Design review of the part built by this model. Coordinates are the model's own, in mm. A direction names the side the tool comes from. Coordinates: 2 decimals unless noted, no trailing zeros. Write each loop counter-clockwise with the first axis right and the second up, starting at its lowest first coordinate (ties: lowest second). Pieces come first, ordered by that corner, then holes.
Q1. For pin 1 Ø5 at (y, z) = (-15, 40.5) entering from +X; pin 2 Ø4 at (x, z) = (-8.5, 45) entering from +Y; pin 3 Ø4 at (y, z) = (-9.06, 89) entering from +X, all flat-tipped, find the tip position at first contact; note any pin that passes through.
Q2. The part is to be moulded in two halves that separate along Z. For faces 1 (the flat face through (-12, -16.564, 48)), 2 (the cylindrical face through (-11.62, -15.82, 87.57)), say which applies: released by +Z, released by -Z, zero draft, split by the parting line, or undercut.
Q3. Take a section at D-D, the plane y = -2.75. Write out the cut boundary in (x, z), plus the area to 3 significant figures.
Q4. Take a section at B-B, the plane y = -9.25. Write out the cut boundary in (x, z).
Q5. For L1, parallel to Y at x = -18.95, z = 89; L2, parallel to X at y = -16, z = 89; L3, parallel to Y at x = -5.75, z = 57.5, list the stretches that pass through material, from the lowest coordinate up.
Q6. Take a section at A-A, the plane z = 7.5. Write out the cut boundary in (x, y).
Q7. Take a section at C-C, the plane x = -15.5. Write out the cut boundary in (y, z), plus the area to 3 significant figures.
Q8. For faces 3 (the flat face through (-4.573, -16, 48)), 4 (the flat face through (-18.073, -8, 48)), list the 3-axis set-ups (+Z, -Z, +X, -X, +Y, -Y) from which the entire face can be reached by the end or side of a thin tool; tool diameter is ignored.
from build123d import *

# Parameters (mm, degrees)
EXTRUSION1_DEPTH = 96.5
ESQUISSE2_R      = 1.5
EXTRUSION2_DEPTH = 98
ESQUISSE3_R      = 1.5
EXTRUSION3_DEPTH = 98


with BuildPart() as part:
    # Esquisse1 → Extrusion1 (new body)
    with BuildSketch(Plane.XY):
        Polygon((-19.573013681, -1.563756614), (-19.573013681, -16.563756614), (-4.573013681, -16.563756614), (-4.573013681, -15.063756614), (-18.073013681, -15.063756614), (-18.073013681, -1.563756614), align=None)
    extrude(amount=EXTRUSION1_DEPTH)

    # Esquisse2 → Extrusion2 (cut)
    with BuildSketch(Plane.XZ.offset(16.563756614)):
        with Locations(Location((-12.073013681, 89, 0), (0, 0, 270))):
            Circle(ESQUISSE2_R)
        with Locations(Location((-12.073013681, 7.5, 0), (0, 0, 270))):
            Circle(ESQUISSE2_R)
    extrude(amount=-EXTRUSION2_DEPTH, mode=Mode.SUBTRACT)

    # Esquisse3 → Extrusion3 (cut)
    with BuildSketch(Plane.ZY.offset(19.573013681)):
        with Locations(Location((89, -9.063756614, 0), (0, 0, 270))):
            Circle(ESQUISSE3_R)
        with Locations(Location((7.5, -9.063756614, 0), (0, 0, 270))):
            Circle(ESQUISSE3_R)
    extrude(amount=-EXTRUSION3_DEPTH, mode=Mode.SUBTRACT)


solid = part.part
Responses:
1. pin 1: stops at x = -4.57
1. pin 2: stops at y = -15.06
1. pin 3: stops at x = -18.07
2. face 1: zero draft
2. face 2: undercut
3. outline: (-19.57, 0) - (-18.07, 0) - (-18.07, 96.5) - (-19.57, 96.5) - close
3. area: 145 mm2
4. outline: (-19.57, 0) - (-18.07, 0) - (-18.07, 6.01) - (-19.57, 6.01) - close; (-19.57, 8.99) - (-18.07, 8.99) - (-18.07, 87.51) - (-19.57, 87.51) - close; (-19.57, 90.49) - (-18.07, 90.49) - (-18.07, 96.5) - (-19.57, 96.5) - close
5. L1: y = -16.56 to -10.56, -7.56 to -1.56
5. L2: x = -19.57 to -13.57, -10.57 to -4.57
5. L3: y = -16.56 to -15.06
6. outline: (-19.57, -16.56) - (-13.57, -16.56) - (-13.57, -15.06) - (-18.07, -15.06) - (-18.07, -10.56) - (-19.57, -10.56) - close; (-19.57, -7.56) - (-18.07, -7.56) - (-18.07, -1.56) - (-19.57, -1.56) - close; (-10.57, -16.56) - (-4.57, -16.56) - (-4.57, -15.06) - (-10.57, -15.06) - close
7. outline: (-16.56, 0) - (-15.06, 0) - (-15.06, 96.5) - (-16.56, 96.5) - close
7. area: 145 mm2
8. face 3: +Z, -Z, +X, +Y, -Y
8. face 4: +Z, -Z, +X, +Y
